Input: part model. Units: mm. Frame: model coordinates. A direction names the side the tool comes from. Give positions to 0.01 mm unless a question says otherwise; leave off trailing zeros. Loops run counter-clockwise (first coordinate to the right, second up) from the corner with the lowest first, then second, coordinate; pieces in that order, holes last. Notation, with made-up numbers: (43.5, 81) -> (65.5, 81) arc R14 cw to (65.5, 89) -> close; hole circle Ø2 at (-26.5, 74). An arc over 180 degrees is marked (long way). Answer as a JSON object with one key per item and string values.
```python
from build123d import *

# Parameters (mm, degrees)
SKETCH1_R           = 2.5
BOSS_EXTRUDE1_DEPTH = 5


with BuildPart() as part:
    # Sketch1 → Boss-Extrude1 (new body)
    with BuildSketch(Plane.XY):
        Polygon((0, 0), (50, 0), (71.213203436, 21.213203436), (60.606601718, 31.819805153), (43.786796564, 15), (0, 15), align=None)
        with Locations((7.5, 7.5)):
            Circle(SKETCH1_R, mode=Mode.SUBTRACT)
    extrude(amount=BOSS_EXTRUDE1_DEPTH)

    # Sketch2 → Revolve2 (revolve)
    with BuildSketch(Plane.XY.offset(2.5)):
        with BuildLine():
            Line((65.909902577, 26.516504294), (85.70209083, 46.308692548))
            ThreePointArc((85.70209083, 46.308692548), (88.085870169, 28.20209083), (71.213203436, 21.213203436))
            Line((71.213203436, 21.213203436), (65.909902577, 26.516504294))
        make_face()
    revolve(axis=Axis((65.909902577, 26.516504294, 2.5), (0.7071067811865461, 0.7071067811865489, 0)))


solid = part.part
```
Q1. Pin query (flat end, axial travel): pin 1 (9.5 mm diameter, centred on x = 34.5, y = 11.5, fed in from +Z); pin 2 (6 mm diameter, centred on x = 7.5, y = 7.5, fed in from -Z); pin 3 (10 mm diameter, centred on x = 62, z = 13.5, fed in from +Y); pin 4 (8 mm diameter, centred on x = 44, y = 25.5, fed in from +Z). Return the tip coordinate at first contact, or that it passes through.
Evaluation:
{"pin 1": "stops at z = 5", "pin 2": "stops at z = 0", "pin 3": "stops at y = 44.56", "pin 4": "passes through"}
Q2. Draft query along X for faces 1 (the cylindrical face through (8.65, 5.28, 2.46)), 2 (the flat face through (52.314, 23.528, 2.465)), 3 (the flat face through (35, 9, 0)). Return one class per face: +X half, -X half, draft (parallel to the pull), parting line (faces both ways), or undercut.
Evaluation:
{"face 1": "undercut", "face 2": "-X half", "face 3": "draft"}
Q3. Section A-A, the plane x = 7.5. Return the cut outline in (y, z), then the cut area to 3 significant figures.
Evaluation:
{"outline": "(0, 0) -> (5, 0) -> (5, 5) -> (0, 5) -> close; (10, 0) -> (15, 0) -> (15, 5) -> (10, 5) -> close", "area": "50.0 mm2"}
Q4. Ray query, line 1 along Y through (x, z) = (7.5, 4.05); line 2 along Z through (x, y) = (55.5, 13.5); line 3 along X through (y, z) = (23.5, 2.5). Return the intervals inside material, ascending.
Evaluation:
{"line 1": "y = 0 to 5, 10 to 15", "line 2": "z = 0 to 5", "line 3": "x = 52.29 to 83.82"}
Q5. Section B-B, the plane x = 25.5. Return the cut outline in (y, z), then the cut area to 3 significant figures.
Evaluation:
{"outline": "(0, 0) -> (15, 0) -> (15, 5) -> (0, 5) -> close", "area": "75.0 mm2"}
Q6. Section C-C, the plane y = 26. Return the cut outline in (x, z), then the cut area to 3 significant figures.
Evaluation:
{"outline": "(54.79, 0) -> (66.43, 0) -> (66.43, -4.96) arc R11.44 ccw (long way) to (66.43, 9.96) -> (66.43, 5) -> (54.79, 5) -> close", "area": "441 mm2"}
Q7. Access query for faces 4 (the flat face through (22, 15, 2)), 5 (the flat face through (65.84, 26.587, -1.979)), 6 (the flat face through (65.84, 26.587, 6.909)), 7 (the flat face through (0, 8, 2)), 8 (the flat face through (25, 0, 2)). Directions: +Z, -Z, +X, -X, +Y, -Y. A direction counts if a zero-diameter tool reaches every point of the face in a straight line with its end or side. Return the directions, or none.
Evaluation:
{"face 4": "+Z, -Z, -X, +Y", "face 5": "-Z, -X, -Y", "face 6": "+Z, -X, -Y", "face 7": "+Z, -Z, -X, +Y, -Y", "face 8": "+Z, -Z, +X, -X, -Y"}
Q8. Section D-D, the plane z = 12.5. Return the cut outline in (x, y), then the cut area to 3 significant figures.
Evaluation:
{"outline": "circle Ø22.36 at (75.1, 35.7)", "area": "393 mm2"}
